Here's how the part is built. I have some questions about the finished solid (model axes, mm). Face numbers are marked on the shaded views. Round coordinates to 2 decimals unless told otherwise and drop trailing zeros. Answer as a JSON object with one key per item and string values.
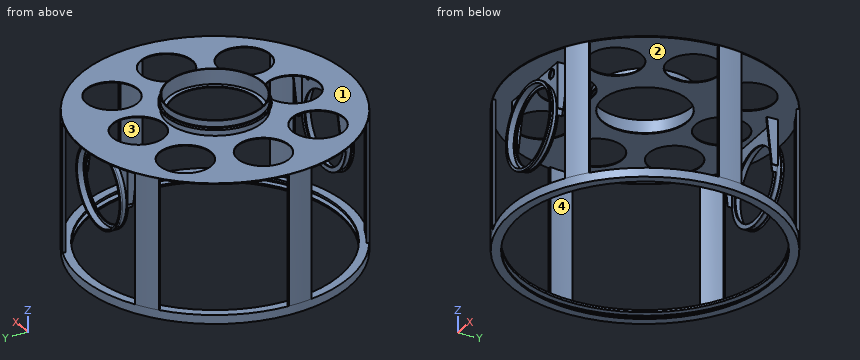
from build123d import *

# Parameters (mm, degrees)
SKETCH1_R                   = 311
SKETCH1_R_2                 = 290.1
EXTRUDE1_DEPTH              = 4
SKETCH3_R                   = 311
SKETCH3_R_2                 = 305
EXTRUDE2_DEPTH              = 11.5
SKETCH4_R                   = 311
SKETCH4_R_2                 = 290.1
EXTRUDE3_DEPTH              = 5
EXTRUDE4_DEPTH              = 300
SKETCH6_R                   = 311
EXTRUDE5_DEPTH              = 2
SKETCH7_R                   = 110.37
SKETCH7_R_2                 = 108.37
EXTRUDE6_DEPTH              = 15
SKETCH8_R                   = 114.4
SKETCH8_R_2                 = 108.37
EXTRUDE7_DEPTH              = 5
SKETCH9_R                   = 110.37
SKETCH9_R_2                 = 108.37
EXTRUDE8_DEPTH              = 15
EXTRUDE9_DEPTH              = 200
SKETCH11_R                  = 90.96
SKETCH11_R_2                = 88.96
EXTRUDE10_DEPTH             = 10
SKETCH13_R                  = 92.96
SKETCH13_R_2                = 88.96
EXTRUDE11_DEPTH             = 5
SKETCH14_R                  = 90.96
SKETCH14_R_2                = 88.96
EXTRUDE12_DEPTH             = 10
SKETCH15_R                  = 94.96
SKETCH15_R_2                = 88.96
EXTRUDE13_DEPTH             = 5
EXTRUDE14_REACH             = 221.04
EXTRUDE14_DIRECTION_2_REACH = 404.96
EXTRUDE15_REACH             = 221.04
EXTRUDE15_DIRECTION_2_REACH = 404.96
SKETCH18_R                  = 11.1125
SKETCH18_R_2                = 82
EXTRUDE16_DEPTH             = 25
SKETCH19_R                  = 11.1125
SKETCH19_R_2                = 82
EXTRUDE18_DEPTH             = 25
SKETCH20_R                  = 98.425
SKETCH20_R_2                = 60
EXTRUDE19_DEPTH             = 2


with BuildPart() as part:
    # Sketch1 → Extrude1 (new body)
    with BuildSketch(Plane.XY):
        Circle(SKETCH1_R)
        Circle(SKETCH1_R_2, mode=Mode.SUBTRACT)
    extrude(amount=EXTRUDE1_DEPTH)

    # Sketch3 → Extrude2 (add)
    with BuildSketch(Plane.XY.offset(4)):
        Circle(SKETCH3_R)
        Circle(SKETCH3_R_2, mode=Mode.SUBTRACT)
    extrude(amount=EXTRUDE2_DEPTH)

    # Sketch4 → Extrude3 (add)
    with BuildSketch(Plane.XY.offset(15.5)):
        Circle(SKETCH4_R)
        Circle(SKETCH4_R_2, mode=Mode.SUBTRACT)
    extrude(amount=EXTRUDE3_DEPTH)

    # Sketch5 → Extrude4 (add)
    with BuildSketch(Plane.XY.offset(20.5)):
        with BuildLine():
            Line((300.366364669, 52.962694188), (306.275211187, 54.004583254))
            ThreePointArc((306.275211187, 54.004583254), (309.816551107, 27.105435995), (311, 0))
            Line((311, 0), (305, 0))
            ThreePointArc((305, 0), (303.839382918, 26.582501538), (300.366364669, 52.962694188))
        make_face()
        with BuildLine():
            Line((152.5, 264.137748154), (155.5, 269.333900577))
            ThreePointArc((155.5, 269.333900577), (131.434279401, 281.861721768), (106.368264574, 292.244405064))
            Line((106.368264574, 292.244405064), (104.316143714, 286.60624934))
            ThreePointArc((104.316143714, 286.60624934), (128.898569831, 276.423875046), (152.5, 264.137748154))
        make_face()
        with BuildLine():
            Line((-152.5, 264.137748154), (-155.5, 269.333900577))
            ThreePointArc((-155.5, 269.333900577), (-178.382271705, 254.756285774), (-199.906946613, 238.23982181))
            Line((-199.906946613, 238.23982181), (-196.050220954, 233.643555151))
            ThreePointArc((-196.050220954, 233.643555151), (-174.940813087, 249.841373508), (-152.5, 264.137748154))
        make_face()
        with BuildLine():
            Line((-305, 0), (-311, 0))
            ThreePointArc((-311, 0), (-309.816551107, -27.105435995), (-306.275211187, -54.004583254))
            Line((-306.275211187, -54.004583254), (-300.366364669, -52.962694188))
            ThreePointArc((-300.366364669, -52.962694188), (-303.839382918, -26.582501538), (-305, 0))
        make_face()
        with BuildLine():
            Line((-152.5, -264.137748154), (-155.5, -269.333900577))
            ThreePointArc((-155.5, -269.333900577), (-131.434279401, -281.861721768), (-106.368264574, -292.244405064))
            Line((-106.368264574, -292.244405064), (-104.316143714, -286.60624934))
            ThreePointArc((-104.316143714, -286.60624934), (-128.898569831, -276.423875046), (-152.5, -264.137748154))
        make_face()
        with BuildLine():
            Line((152.5, -264.137748154), (155.5, -269.333900577))
            ThreePointArc((155.5, -269.333900577), (178.382271705, -254.756285774), (199.906946613, -238.23982181))
            Line((199.906946613, -238.23982181), (196.050220954, -233.643555151))
            ThreePointArc((196.050220954, -233.643555151), (174.940813087, -249.841373508), (152.5, -264.137748154))
        make_face()
    extrude(amount=EXTRUDE4_DEPTH)

    # Sketch6 → Extrude5 (add)
    with BuildSketch(Plane.XY.offset(320.5)):
        Circle(SKETCH6_R)
    extrude(amount=EXTRUDE5_DEPTH)

    # Sketch7 → Extrude6 (add)
    with BuildSketch(Plane.XY.offset(322.5)):
        Circle(SKETCH7_R)
        Circle(SKETCH7_R_2, mode=Mode.SUBTRACT)
    extrude(amount=EXTRUDE6_DEPTH)

    # Sketch8 → Extrude7 (add)
    with BuildSketch(Plane.XY.offset(337.5)):
        Circle(SKETCH8_R)
        Circle(SKETCH8_R_2, mode=Mode.SUBTRACT)
    extrude(amount=EXTRUDE7_DEPTH)

    # Sketch9 → Extrude8 (add)
    with BuildSketch(Plane.XY.offset(342.5)):
        Circle(SKETCH9_R)
        Circle(SKETCH9_R_2, mode=Mode.SUBTRACT)
    extrude(amount=EXTRUDE8_DEPTH)

    # Sketch10 → Extrude9 (add)
    with BuildSketch(Plane(origin=(0, 0, 320.5), x_dir=(-1, 0, 0), z_dir=(0, 0, -1))):
        Polygon((94.96, 250), (94.96, 228), (91.96, 228), (91.96, 250), (-91.96, 250), (-91.96, 228), (-94.96, 228), (-94.96, 250), (-94.96, 253), (0, 253), (94.96, 253), align=None)
        Polygon((94.96, -250), (94.96, -228), (91.96, -228), (91.96, -250), (-91.96, -250), (-91.96, -228), (-94.96, -228), (-94.96, -250), (-94.96, -253), (94.96, -253), align=None)
    extrude(amount=EXTRUDE9_DEPTH)

    # Sketch11 → Extrude10 (add)
    with BuildSketch(Plane(origin=(0, 253, 0), x_dir=(1, 0, 0), z_dir=(0, 1, 0))):
        with Locations((0.393539239, -215.46)):
            Circle(SKETCH11_R)
        with Locations((0.393539239, -215.46)):
            Circle(SKETCH11_R_2, mode=Mode.SUBTRACT)
    extrude(amount=EXTRUDE10_DEPTH)

    # Sketch13 → Extrude11 (add)
    with BuildSketch(Plane(origin=(0, 263, 0), x_dir=(1, 0, 0), z_dir=(0, 1, 0))):
        with Locations((0.393539239, -215.46)):
            Circle(SKETCH13_R)
        with Locations((0.393539239, -215.46)):
            Circle(SKETCH13_R_2, mode=Mode.SUBTRACT)
    extrude(amount=EXTRUDE11_DEPTH)

    # Sketch14 → Extrude12 (add)
    with BuildSketch(Plane.XZ.offset(253)):
        with Locations((0, 215.46)):
            Circle(SKETCH14_R)
        with Locations((0, 215.46)):
            Circle(SKETCH14_R_2, mode=Mode.SUBTRACT)
    extrude(amount=EXTRUDE12_DEPTH)

    # Sketch15 → Extrude13 (add)
    with BuildSketch(Plane.XZ.offset(263)):
        with Locations((0, 215.46)):
            Circle(SKETCH15_R)
        with Locations((0, 215.46)):
            Circle(SKETCH15_R_2, mode=Mode.SUBTRACT)
    extrude(amount=EXTRUDE13_DEPTH)

    # Extrude14: up to this face of the body (flat: up to its plane)
    extrude14_end = Plane(part.part.faces().sort_by_distance((94.96, 240.5, 220.5))[0])
    # Sketch16 → Extrude14 (cut, up to the picked face)
    with BuildSketch(Plane.ZY.offset(-91.96), mode=Mode.PRIVATE) as extrude14_sk1:
        Polygon((120.5, 228), (320.5, 228), (120.5, 250), align=None)
    extrude14_tool1 = split(extrude(extrude14_sk1.sketch, amount=-EXTRUDE14_REACH, mode=Mode.PRIVATE), bisect_by=extrude14_end, keep=Keep.BOTH, mode=Mode.PRIVATE)
    add(extrude14_tool1.solids().sort_by_distance((91.96, 235.333333, 187.166667))[0], mode=Mode.SUBTRACT)

    # Extrude14 direction 2: up to this face of the body (flat: up to its plane)
    extrude14_direction_2_end = Plane(part.part.faces().sort_by_distance((-94.96, 240.5, 220.5))[0])
    # Sketch16 → Extrude14 direction 2 (cut, up to the picked face)
    with BuildSketch(Plane.ZY.offset(-91.96), mode=Mode.PRIVATE) as extrude14_direction_2_sk1:
        Polygon((120.5, 228), (320.5, 228), (120.5, 250), align=None)
    extrude14_direction_2_tool1 = split(extrude(extrude14_direction_2_sk1.sketch, amount=EXTRUDE14_DIRECTION_2_REACH, mode=Mode.PRIVATE), bisect_by=extrude14_direction_2_end, keep=Keep.BOTH, mode=Mode.PRIVATE)
    add(extrude14_direction_2_tool1.solids().sort_by_distance((91.96, 235.333333, 187.166667))[0], mode=Mode.SUBTRACT)

    # Extrude15: up to this face of the body (flat: up to its plane)
    extrude15_end = Plane(part.part.faces().sort_by_distance((-94.96, -240.5, 220.5))[0])
    # Sketch17 → Extrude15 (cut, up to the picked face)
    with BuildSketch(Plane(origin=(-91.96, 0, 0), x_dir=(0, 0, -1), z_dir=(1, 0, 0)), mode=Mode.PRIVATE) as extrude15_sk1:
        Polygon((-320.5, -228), (-120.5, -228), (-120.5, -250), align=None)
    extrude15_tool1 = split(extrude(extrude15_sk1.sketch, amount=-EXTRUDE15_REACH, mode=Mode.PRIVATE), bisect_by=extrude15_end, keep=Keep.BOTH, mode=Mode.PRIVATE)
    add(extrude15_tool1.solids().sort_by_distance((-91.96, -235.333333, 187.166667))[0], mode=Mode.SUBTRACT)

    # Extrude15 direction 2: up to this face of the body (flat: up to its plane)
    extrude15_direction_2_end = Plane(part.part.faces().sort_by_distance((94.96, -240.5, 220.5))[0])
    # Sketch17 → Extrude15 direction 2 (cut, up to the picked face)
    with BuildSketch(Plane(origin=(-91.96, 0, 0), x_dir=(0, 0, -1), z_dir=(1, 0, 0)), mode=Mode.PRIVATE) as extrude15_direction_2_sk1:
        Polygon((-320.5, -228), (-120.5, -228), (-120.5, -250), align=None)
    extrude15_direction_2_tool1 = split(extrude(extrude15_direction_2_sk1.sketch, amount=EXTRUDE15_DIRECTION_2_REACH, mode=Mode.PRIVATE), bisect_by=extrude15_direction_2_end, keep=Keep.BOTH, mode=Mode.PRIVATE)
    add(extrude15_direction_2_tool1.solids().sort_by_distance((-91.96, -235.333333, 187.166667))[0], mode=Mode.SUBTRACT)

    # Sketch18 → Extrude16 (cut)
    with BuildSketch(Plane(origin=(0, 253, 0), x_dir=(1, 0, 0), z_dir=(0, 1, 0))):
        with Locations((69.85, -304.8)):
            Circle(SKETCH18_R)
        with Locations((-69.85, -304.8)):
            Circle(SKETCH18_R)
        with Locations((0.393539239, -215.46)):
            Circle(SKETCH18_R_2)
        with BuildLine():
            Line((93.173539239, -215.46), (94.96, -215.46))
            Line((94.96, -215.46), (94.96, -120.5))
            Line((94.96, -120.5), (-94.96, -120.5))
            Line((-94.96, -120.5), (-94.96, -215.46))
            Line((-94.96, -215.46), (-92.386460761, -215.46))
            ThreePointArc((-92.386460761, -215.46), (0.393539239, -122.68), (93.173539239, -215.46))
        make_face()
    extrude(amount=-EXTRUDE16_DEPTH, mode=Mode.SUBTRACT)

    # Sketch19 → Extrude18 (cut)
    with BuildSketch(Plane.XZ.offset(253)):
        with Locations((69.85, 304.8)):
            Circle(SKETCH19_R)
        with Locations((-69.85, 304.8)):
            Circle(SKETCH19_R)
        with Locations((0.393539239, 215.46)):
            Circle(SKETCH19_R_2)
        with BuildLine():
            Line((93.173539239, 215.46), (94.96, 215.46))
            Line((94.96, 215.46), (94.96, 120.5))
            Line((94.96, 120.5), (-94.96, 120.5))
            Line((-94.96, 120.5), (-94.96, 215.46))
            Line((-94.96, 215.46), (-92.386460761, 215.46))
            ThreePointArc((-92.386460761, 215.46), (0.393539239, 122.68), (93.173539239, 215.46))
        make_face()
    extrude(amount=-EXTRUDE18_DEPTH, mode=Mode.SUBTRACT)

    # Sketch20 → Extrude19 (cut)
    with BuildSketch(Plane.XY.offset(322.5)):
        Circle(SKETCH20_R)
        with Locations((203.2, 0)):
            Circle(SKETCH20_R_2)
        with Locations((150.8125, 153.9875)):
            Circle(SKETCH20_R_2)
        with Locations((-3.175, 177.8)):
            Circle(SKETCH20_R_2)
        with Locations((-153.9875, 152.4)):
            Circle(SKETCH20_R_2)
        with Locations((-203.2, 0)):
            Circle(SKETCH20_R_2)
        with Locations((-153.9875, -152.4)):
            Circle(SKETCH20_R_2)
        with Locations((0, -179.3875)):
            Circle(SKETCH20_R_2)
        with Locations((152.4, -150.8125)):
            Circle(SKETCH20_R_2)
    extrude(amount=-EXTRUDE19_DEPTH, mode=Mode.SUBTRACT)


solid = part.part
Item 1: Please list where these lines run through material, in increasing order: probe 1 along Y at (x, z) = (0, 18.3); probe 2 along Y at (x, z) = (0, 321) (1 decimal); probe 3 along X at (y, z) = (-152, 321). Write a range as from..to.
Resolved:
{"probe 1": "-311..-290.1, 290.1..311", "probe 2": "-311..-239.4, -119.4..-98.4, 98.4..117.9, 237.7..311", "probe 3": "-271.32..-213.99, -93.99..-53.38, 53.38..92.41, 212.39..271.32"}
Item 2: If we mould it in two halves opening along Y, with no side actions, what happens to the marked faces 1, 2, 3 and 4? For each: pulls with the +Y half, pulls with the -Y half, needs draft (parallel to the pull), parting line crosses it, or undercut.
Resolved:
{"face 1": "needs draft", "face 2": "undercut", "face 3": "pulls with the -Y half", "face 4": "pulls with the +Y half"}
Item 3: I'm going to push flat-ended pins straight in: pin 1 Ø7.5 at (y, z) = (-240.5, 247) entering from +X; pin 2 Ø7.5 at (y, z) = (240.5, 286) entering from -X; pin 3 Ø2 at (y, z) = (49.5, 92.5) entering from -X. Where does each tip first touch, or does it pass through?
Resolved:
{"pin 1": "x = 199.91", "pin 2": "x = -199.91", "pin 3": "x = 300.79"}
Item 4: I want a section at A-A, the plane y = 192. State how many separate pieces and enclosed holes the cut face has, then the cut area to 3 significant figures.
Resolved:
{"separate pieces": "6", "enclosed holes": "0", "area": "1,050 mm²"}
